from build123d import *

# Parameters (mm, degrees)
F0_W     = 52.5
F0_H     = 60
F1_DEPTH = 20
F3_DEPTH = 25
F4_R     = 2.5


with BuildPart() as f1:
    # F0 (on Front) → F1 (new body)
    with BuildSketch(Plane.XZ):
        with Locations((26.25, 30)):
            Rectangle(F0_W, F0_H)
        with Locations((-26.25, 30)):
            Rectangle(F0_W, F0_H)
    extrude(amount=F1_DEPTH)

    # F2 (on Front) → F3 (cut)
    with BuildSketch(Plane.XZ):
        with BuildLine():
            ThreePointArc((7.5, 30), (5.303301, 35.303301), (0, 37.5))
            Line((0, 37.5), (0, 30))
            Line((0, 30), (7.5, 30))
        make_face()
        with BuildLine():
            ThreePointArc((32.5, 30), (25, 37.5), (17.5, 30))
            Line((17.5, 30), (25, 30))
            Line((25, 30), (32.5, 30))
        make_face()
        with BuildLine():
            Line((25, 30), (17.5, 30))
            ThreePointArc((17.5, 30), (25, 22.5), (32.5, 30))
            Line((32.5, 30), (25, 30))
        make_face()
        with BuildLine():
            ThreePointArc((-32.5, 30), (-25, 22.5), (-17.5, 30))
            Line((-17.5, 30), (-25, 30))
            Line((-25, 30), (-32.5, 30))
        make_face()
        with BuildLine():
            Line((-25, 30), (-17.5, 30))
            ThreePointArc((-17.5, 30), (-25, 37.5), (-32.5, 30))
            Line((-32.5, 30), (-25, 30))
        make_face()
        with BuildLine():
            Line((0, 30), (0, 37.5))
            ThreePointArc((0, 37.5), (-5.303301, 35.303301), (-7.5, 30))
            Line((-7.5, 30), (0, 30))
        make_face()
        with BuildLine():
            Line((7.5, 30), (0, 30))
            Line((0, 30), (0, 22.5))
            ThreePointArc((0, 22.5), (5.303301, 24.696699), (7.5, 30))
        make_face()
        with BuildLine():
            Line((0, 22.5), (0, 30))
            Line((0, 30), (-7.5, 30))
            ThreePointArc((-7.5, 30), (-5.303301, 24.696699), (0, 22.5))
        make_face()
    extrude(amount=F3_DEPTH, mode=Mode.SUBTRACT)

    # F4
    f4_edges = [f1.edges().sort_by_distance(p)[0] for p in [
        (52.5, -10, 60),
        (0, -20, 60),
        (-52.5, -10, 60),
        (0, 0, 60),
        (52.5, -10, 0),
        (52.5, 0, 30),
        (52.5, -20, 30),
        (0, 0, 0),
        (-52.5, -10, 0),
        (0, -20, 0),
        (-52.5, 0, 30),
        (-52.5, -20, 30),
    ]]
    fillet(f4_edges, radius=F4_R)


solid = f1.part
The model under review builds one solid part; all positions refer to its coordinate system, in mm. Coordinates: 2 decimals unless noted, no trailing zeros. Loops run counter-clockwise (first coordinate to the right, second up) from the corner with the lowest first, then second, coordinate; pieces in that order, holes last. Notation, with made-up numbers: M 83,-30 L 93,-30 A17 cw 93,0 Z; hole C -10,51.5 d9. An arc over 180 degrees is marked long. Put each result on its own line as item: value. Start each with the question number.
Q1. Add section A-A (x = -4.5). Write out the cut boundary in (y, z), and give its area (3 significant figures).
Q2. Add section C-C (x = -25). Write out the cut boundary in (y, z), and give its area (3 significant figures).
Q3. Clearance check with a flat-ended pin moving along its axis: pin 1 (13.5 mm diameter, centred on x = -25, z = 30, fed in from +Y). State where the tip first meets the part, or that it passes through.
Q4. Add section B-B (y = -13). Write out the cut boundary in (x, z), and give its area (3 significant figures).
Q5. Wall thickness on line 1 (X direction, y = -5.5, z = 30); line 2 (X direction, y = -8.5, z = 35.5); line 3 (Z direction, x = 25, y = -13): over which ranges is each line inside the solid? List them lowest first.
Q6. The part is to be moulded in two halves that separate along Z. For faces 1 (the cylindrical face through (-0.7, -19.248, 59.287)), 2 (the cylindrical face through (30.952, -9.86, 34.564)), 3 (the cylindrical face through (-52, -19, 30)), 4 (the cylindrical face through (-30.952, -9.86, 25.436)), say which applies: +Z half, -Z half, draft (parallel to the pull), parting line (faces both ways), or undercut.
Answers:
1. outline: M -20,2.5 A2.5 ccw -17.5,0 L -2.5,0 A2.5 ccw 0,2.5 L 0,24 L -20,24 Z; M -20,36 L 0,36 L 0,57.5 A2.5 ccw -2.5,60 L -17.5,60 A2.5 ccw -20,57.5 Z
1. area: 955 mm^2
2. outline: M -20,2.5 A2.5 ccw -17.5,0 L -2.5,0 A2.5 ccw 0,2.5 L 0,22.5 L -20,22.5 Z; M -20,37.5 L 0,37.5 L 0,57.5 A2.5 ccw -2.5,60 L -17.5,60 A2.5 ccw -20,57.5 Z
2. area: 895 mm^2
3. pin 1: passes through
4. outline: M -52.5,2.5 A2.5 ccw -50,0 L 50,0 A2.5 ccw 52.5,2.5 L 52.5,57.5 A2.5 ccw 50,60 L -50,60 A2.5 ccw -52.5,57.5 Z; hole C -25,30 d15; hole C 0,30 d15; hole C 25,30 d15
4. area: 5,760 mm^2
5. line 1: x = -52.5 to -32.5, -17.5 to -7.5, 7.5 to 17.5, 32.5 to 52.5
5. line 2: x = -52.5 to -30.1, -19.9 to -5.1, 5.1 to 19.9, 30.1 to 52.5
5. line 3: z = 0 to 22.5, 37.5 to 60
6. face 1: +Z half
6. face 2: undercut
6. face 3: draft
6. face 4: undercut
